For this review, take the finished solid that the model builds, in its own axes (mm). Face numbers are marked on the shaded views. A direction names the side the tool comes from. Give positions to 0.01 mm unless a question says otherwise; leave off trailing zeros. Write each loop counter-clockwise with the first axis right and the second up, starting at its lowest first coordinate (ties: lowest second). Pieces come first, ordered by that corner, then holes. Notation, with made-up numbers: M -27.75,83 L 19.25,83 A27 ccw 19.25,115 Z; hole C -1.75,14.5 d2. An arc over 180 degrees is marked long. Use one line per item in the form item = value. Start each with the question number.
Q1. Tool access review of the marked faces 1 and 2: name each direction out of +Z, -Z, +X, -X, +Y, -Y from which nothing blocks a thin tool from reaching the whole face with its end or side.
Q2. Consider section C-C on z = 63. Write out the cut boundary in (x, y).
Q3. Consider section A-A on y = 0. Write out the cut boundary in (x, z).
Q4. For probe 1 along Y at (x, z) = (0, 1.95); probe 2 along Z at (x, y) = (-10.5, -12); probe 3 along Y at (x, z) = (-8.5, 15), list the stretches that pass through material, from the lowest coordinate up. Write a range as [from, to].
Q5. Clearance check with flat-ended pins moving along their axes: pin 1 Ø6.5 at (x, y) = (0.5, 0) entering from -Z; pin 2 Ø12 at (x, z) = (4, 11.5) entering from +Y; pin 3 Ø6 at (x, z) = (-11.5, 10) entering from -Y; pin 4 Ø5 at (y, z) = (-7, 67) entering from +X. State where each tip first meets the part, or that it passes through.
```python
from build123d import *

# Parameters (mm, degrees)
ESQUISSE1_R             = 29
BOSS_EXTRU_1_DEPTH      = 30
ESQUISSE2_R             = 4
BOSS_EXTRU_2_DEPTH      = 10
ESQUISSE3_R             = 5
BOSS_EXTRU_3_DEPTH      = 3
ESQUISSE4_R             = 4
ENL_V_MAT_EXTRU_1_DEPTH = 5
CHANFREIN1_SIZE         = 1
ESQUISSE8_R             = 4
BOSS_EXTRU_4_DEPTH      = 38
CONG_1_R                = 1


with BuildPart() as part:
    # Esquisse1 → Boss.-Extru.1 (new body)
    with BuildSketch(Plane.XY):
        Circle(ESQUISSE1_R)
    extrude(amount=BOSS_EXTRU_1_DEPTH)

    # Esquisse2 → Boss.-Extru.2 (add)
    with BuildSketch(Plane.XY.offset(30)):
        Circle(ESQUISSE2_R)
    extrude(amount=BOSS_EXTRU_2_DEPTH)

    # Esquisse3 → Boss.-Extru.3 (add)
    with BuildSketch(Plane.XY.offset(30)):
        Circle(ESQUISSE3_R)
    extrude(amount=BOSS_EXTRU_3_DEPTH)

    # Esquisse4 → Enlèv. mat.-Extru.1 (cut)
    with BuildSketch(Plane(origin=(0, 0, 0), x_dir=(-1, 0, 0), z_dir=(0, 0, -1))):
        with Locations(Location((0, 0, 0), (0, 0, 180))):
            Circle(ESQUISSE4_R)
    extrude(amount=-ENL_V_MAT_EXTRU_1_DEPTH, mode=Mode.SUBTRACT)

    # Chanfrein1
    chanfrein1_edges = [part.edges().sort_by_distance(p)[0] for p in [
        (-29, 0, 0),
        (-29, 0, 30),
    ]]
    chamfer(chanfrein1_edges, length=CHANFREIN1_SIZE)

    # Esquisse8 → Boss.-Extru.4 (add)
    with BuildSketch(Plane.XY.offset(40)):
        Circle(ESQUISSE8_R)
    extrude(amount=BOSS_EXTRU_4_DEPTH)

    # Congé1
    cong_1_edges = [part.edges().sort_by_distance(p)[0] for p in [
        (-4, 0, 78),
    ]]
    fillet(cong_1_edges, radius=CONG_1_R)


solid = part.part
```
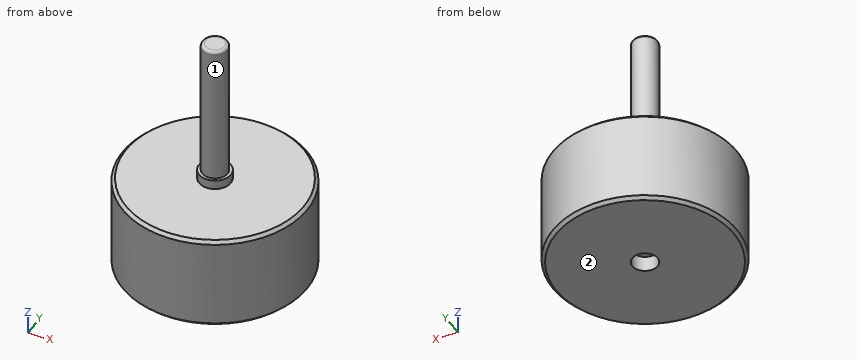
Working result:
q1.face_1 = +Z
q1.face_2 = -Z, +X, -X, +Y, -Y
q2.outline = C 0,0 d8
q3.outline = M -29,1 L -28,0 L -4,0 L -4,5 L 4,5 L 4,0 L 28,0 L 29,1 L 29,29 L 28,30 L 5,30 L 5,33 L 4,33 L 4,77 A1 ccw 3,78 L -3,78 A1 ccw -4,77 L -4,33 L -5,33 L -5,30 L -28,30 L -29,29 Z
q4.probe_1 = [-29, -4], [4, 29]
q4.probe_2 = [0, 30]
q4.probe_3 = [-27.73, 27.73]
q5.pin_1 = 5
q5.pin_2 = 29
q5.pin_3 = -27.73
q5.pin_4 = through
